Here's how the part is built. I have some questions about the finished solid (model axes, mm). A direction names the side the tool comes from. Give positions to 0.01 mm unless a question says otherwise; leave off trailing zeros. Order: outer loops, then holes, each group sorted by start corner. A loop starts at its lowest first (then second) coordinate and runs counter-clockwise, first axis right, second up.
from build123d import *

# Parameters (mm, degrees)
F0_R        = 1.225
F1_DEPTH    = 2.75
F3_DEPTH    = 1.75
F4_W        = 2.8751536738
F4_H        = 5.9757605195
F5_DEPTH    = 13
F6_T1_DEPTH = 3.5
F7_R        = 1
F9_R        = 1.7
F10_DEPTH   = 2.5
F11_DEPTH   = 7.5


# Not quite as in the source:
# - a fillet or chamfer that OpenCascade refuses, or shapes differently, is made with other operations: its cross-section is extruded or revolved along the edge and cut away or added


with BuildPart() as f1:
    # F0 (on Front) → F1 (new body, symmetric)
    with BuildSketch(Plane.XZ):
        with BuildLine():
            Line((-2.7517704794, 0.9889971563), (2.7379837894, 2.1785584332))
            Line((2.7379837894, 2.1785584332), (2.4390654013, 36.1785584332))
            ThreePointArc((2.4390654013, 36.1785584332), (-0.3350046134, 38.9042758715), (-3.0607220517, 36.1302058568))
            Line((-3.0607220517, 36.1302058568), (-2.7517704794, 0.9889971563))
        make_face()
        with BuildLine():
            Line((-1.3813343576, 5.0087761541), (-1.3813707205, 32.1587761541))
            ThreePointArc((-1.3813707205, 32.1587761541), (-0.1563723611, 33.3837777948), (1.0686292795, 32.1587794355))
            Line((1.0686292795, 32.1587794355), (1.0686656424, 5.0087794355))
            ThreePointArc((1.0686656424, 5.0087794355), (-0.1563327169, 3.7837777948), (-1.3813343576, 5.0087761541))
        make_face(mode=Mode.SUBTRACT)
        with Locations((-0.3108283252, 36.154382145)):
            Circle(F0_R, mode=Mode.SUBTRACT)
    extrude(amount=F1_DEPTH, both=True)

    # F2 (on Front) → F3 (join, symmetric)
    with BuildSketch(Plane.XZ):
        Polygon((-2.9082125786, 27.7813646846), (-2.9082125786, 33.2853169523), (-5.5837442831, 33.2853169523), (-5.5837442831, 8.1353169523), (-3.9784252097, 8.1353169523), (-3.9784252097, 12.1868369773), (-3.9784252097, 27.7813646846), align=None)
        with BuildLine():
            Line((-3.9784252097, 12.1868369773), (-3.9784252097, 8.1353169523))
            ThreePointArc((-3.9784252097, 8.1353169523), (-3.0542834819, 10.1610769648), (-3.9784252097, 12.1868369773))
        make_face()
    extrude(amount=F3_DEPTH, both=True)

    # F4 (on Right) → F5 (cut, symmetric)
    with BuildSketch(Plane.YZ):
        with Locations((0, 37.1919497848)):
            Rectangle(F4_W, F4_H)
    extrude(amount=F5_DEPTH, both=True, mode=Mode.SUBTRACT)

    # F6: fillet of radius 1 on 1 edges, made by hand

    # F6_s2 → F6_t1 (join)
    with BuildSketch(Plane.XZ.offset(-1.75)):
        with BuildLine():
            ThreePointArc((-2.9784252097, 27.7813646846), (-3.6855319909, 27.4884714657), (-3.9784252097, 26.7813646846))
            Line((-3.9784252097, 26.7813646846), (-3.9784252097, 27.7813646846))
            Line((-3.9784252097, 27.7813646846), (-2.9784252097, 27.7813646846))
        make_face()
    extrude(amount=F6_T1_DEPTH)

    # F7
    f7_edges = [f1.edges().sort_by_distance(p)[0] for p in [
        (-5.583744, 0, 33.285317),
        (-4.781085, 1.75, 8.135317),
        (-4.781085, -1.75, 8.135317),
    ]]
    fillet(f7_edges, radius=F7_R)

    # F9 (on offset) → F10 (join)
    with BuildSketch(Plane(origin=(-0.3281029821, 0, 1.5141756728), x_dir=(0.9773189207, 0, 0.2117728201), z_dir=(0.2117728201, 0, -0.9773189207))):
        Polygon((2.0697711183, -2.2267070605), (3.3573344565, -0.0034180592), (2.0756913705, 2.2232890013), (-0.4935150537, 2.2267070605), (-1.7810783919, 0.0034180592), (-0.4994353059, -2.2232890013), align=None)
        with Locations((0.7881280323, 0)):
            Circle(F9_R, mode=Mode.SUBTRACT)
    extrude(amount=F10_DEPTH)

    # F11 (add): a face of the model
    f11_faces = [f1.faces().sort_by_distance(p)[0] for p in [
        (0.4421494557, 0, 1.6810797688),
    ]]
    extrude(f11_faces, amount=F11_DEPTH)


solid = f1.part
Q1. I'm going to push flat-ended pins straight in: P1, Ø1.3, axis at x = -4.5, z = 22, coming from the +Y side; P2, Ø2, axis at x = -0.31, z = 36.15, coming from the +Y side; P3, Ø0.9, axis at x = -0.5, y = 0.5, coming from the +Z side; P4, Ø0.5, axis at x = -4, y = 0.5, coming from the +Z side. Where does each tip first touch, or does it pass through?
Filled sheet:
P1: stops at y = 1.75
P2: passes through
P3: stops at z = 34.2
P4: stops at z = 33.29
Q2. I need wall thicknesses on L1, parallel to X at y = -0.2, z = 27.5; L2, parallel to X at y = 1.45, z = 14; L3, parallel to Z at x = -1, y = 2.35. Which ranges of each line are inside material? Lowest first, please.
Filled sheet:
L1: x = -5.58 to -3.67, -2.98 to -1.38, 1.07 to 2.52
L2: x = -5.58 to -3.98, -2.87 to -1.38, 1.07 to 2.63
L3: z = 1.37 to 4.12, 33.05 to 35.14, 37.17 to 38.82
Q3. For faces 1 (the face through (2.576, 1.131, 0.882)), 2 (the face through (-4.66, -1.45, 8.42)), 3 (the face through (-4.66, 1.45, 8.42)), which set-ups out of +Z, -Z, +X, -X, +Y, -Y let a thin tool reach every point of the face, with its end or its side?
Filled sheet:
face 1: +X, +Y
face 2: -Z, -X, -Y
face 3: -Z, -X, +Y
Q4. If we section it at A-A on z = 6.5: List the corners of the cut face in (x, y) for me.
Filled sheet:
outline: (-2.8, -2.75) - (-1.38, -2.75) - (-1.38, 2.75) - (-2.8, 2.75) - close; (1.07, -2.75) - (2.7, -2.75) - (2.7, 2.75) - (1.07, 2.75) - close
Q5. If we section it at B-B on z = 19.5: List the corners of the cut face in (x, y) for me.
Filled sheet:
outline: (-5.58, -1.75) - (-3.98, -1.75) - (-3.98, 1.75) - (-5.58, 1.75) - close; (-2.91, -2.75) - (-1.38, -2.75) - (-1.38, 2.75) - (-2.91, 2.75) - close; (1.07, -2.75) - (2.59, -2.75) - (2.59, 2.75) - (1.07, 2.75) - close
Q6. Thinking about a two-plate mould opening in X: for faces 4 (the face through (-5.283, -0.024, 33)), 5 (the face through (-0.275, -2.103, 38.904)), 6 (the face through (-3.978, 0, 19)), 7 (the face through (0, 0, 34.204)), which applies, released by +X, released by -X, zero draft, split by the parting line, or undercut?
Filled sheet:
face 4: released by -X
face 5: split by the parting line
face 6: undercut
face 7: zero draft
Q7. If we section it at D-D on x = -5: List the corners of the cut face in (y, z) for me.
Filled sheet:
outline: (-1.75, 9.14) arc R1 ccw to (-0.75, 8.14) - (0.75, 8.14) arc R1 ccw to (1.75, 9.14) - (1.75, 33.19) - (-1.75, 33.19) - close
Q8. If we section it at C-C on z = 35.5: List the corners of the cut face in (x, y) for me.
Filled sheet:
outline: (-3.06, -2.75) - (-1.35, -2.75) - (-1.35, -1.44) - (-3.06, -1.44) - close; (-3.06, 1.44) - (-1.35, 1.44) - (-1.35, 2.75) - (-3.06, 2.75) - close; (0.72, -2.75) - (2.45, -2.75) - (2.45, -1.44) - (0.72, -1.44) - close; (0.72, 1.44) - (2.45, 1.44) - (2.45, 2.75) - (0.72, 2.75) - close
